For this review, take the finished solid that the model builds, in its own axes (mm). Give positions to 0.01 mm unless a question says otherwise; leave off trailing zeros. Write each loop counter-clockwise with the first axis right and the second up, starting at its lowest first coordinate (ties: lowest second). Pieces come first, ordered by that corner, then holes.
1) For P1, Ø3, axis at x = 31, z = 2.5, coming from the -Y side; P2, Ø3, axis at x = 5, y = -4.5, coming from the -Z side, all flat-tipped, find the tip position at first contact; note any pin that passes through.
2) Wall thickness on line 1 along X through (y, z) = (-14.25, 0.5); line 2 along Y through (x, z) = (17, 3.6); line 3 along Z through (x, y) = (31, -18.5): over which ranges is each line inside the solid? List them lowest first.
3) We need section C-C on y = -14.5. Give the boundary of the cut face in (x, z).
4) We need section A-A on z = 2.5. Give the boundary of the cut face in (x, y).
5) We need section B-B on x = 17. Give the boundary of the cut face in (y, z).
6) We need section D-D on x = 3. Give the boundary of the cut face in (y, z).
Autodesk Fusion 360 part; units mm, degrees
sketch "Sketch1" plane through (0, 0, 0) normal (0, 0, 1) x (1, 0, 0)
  line L0 (0, 0) -> (34, 0)
  line L1 (34, 0) -> (34, -29)
  line L2 (34, -29) -> (0, -29)
  line L3 (0, -29) -> (0, 0)
  circle A0 centre (17, -14.5) radius 11
  dimension "d1" = 34
  dimension "d2" = 29
  dimension "d3" = 22
extrude "Extrude1" add sketch "Sketch1" along normal blind 5
sketch "Sketch2" plane through (0, 0, 0) normal (0, 1, 0) x (1, 0, 0)
  circle A0 centre (3, -2.5) radius 1.7
  circle A1 centre (31, -2.5) radius 1.7
  dimension "d6" = 3.4
  dimension "d7" = 3.4
extrude "Extrude2" cut sketch "Sketch2" against normal blind 29
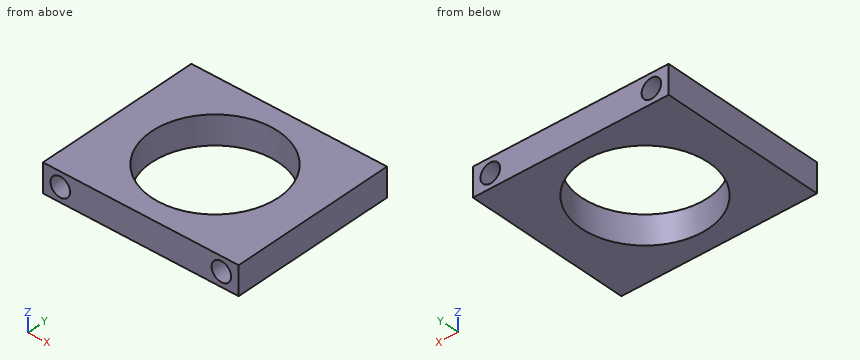
Results list:
1. P1: passes through
1. P2: stops at z = 0
2. line 1: x = 0 to 6, 28 to 34
2. line 2: y = -29 to -25.5, -3.5 to 0
2. line 3: z = 0 to 0.8, 4.2 to 5
3. outline: (0, 0) - (6, 0) - (6, 5) - (0, 5) - close; (28, 0) - (34, 0) - (34, 5) - (28, 5) - close; hole circle Ø3.4 at (3, 2.5); hole circle Ø3.4 at (31, 2.5)
4. outline: (0, -29) - (1.3, -29) - (1.3, 0) - (0, 0) - close; (4.7, -29) - (29.3, -29) - (29.3, 0) - (4.7, 0) - close; (32.7, -29) - (34, -29) - (34, 0) - (32.7, 0) - close; hole circle Ø22 at (17, -14.5)
5. outline: (-29, 0) - (-25.5, 0) - (-25.5, 5) - (-29, 5) - close; (-3.5, 0) - (0, 0) - (0, 5) - (-3.5, 5) - close
6. outline: (-29, 0) - (0, 0) - (0, 0.8) - (-29, 0.8) - close; (-29, 4.2) - (0, 4.2) - (0, 5) - (-29, 5) - close
